Build history of the part. All positions in model axes, mm. A direction names the side the tool comes from. Give positions to 0.01 mm unless a question says otherwise; leave off trailing zeros. Write each loop counter-clockwise with the first axis right and the second up, starting at its lowest first coordinate (ties: lowest second). Pieces come first, ordered by that corner, then holes. Notation, with made-up numbers: (59.25, 23.5) -> (106.25, 23.5) arc R23 cw to (106.25, 43.5) -> close; hole circle Ø7 at (4.25, 34). An arc over 180 degrees is marked (long way). Write item = value, one per line. Start each with the question number.
Q1. Saw through at B-B, the plane z = 0. Give the number of separate pieces and of enclosed holes in the cut face, then the cut area to 3 significant figures.
Q2. Mould opens along Z. For faces 1 (the face through (49, 5, -11.8)), 2 (the face through (45, 9, 6)), 3 (the face through (-29, 10, -7)) say: pulls with the +Z half, pulls with the -Z half, needs draft (parallel to the pull), parting line crosses it, or undercut.
Q3. Wall check: line 1 (Z direction, x = 19, y = 6); line 2 (Z direction, x = -8, y = 9.75); line 3 (X direction, y = 7.75, z = -10.5). Give the ranges that are in metal, low to high.
Q4. Drop flat-ended pins along their axis: P1, Ø2, axis at x = 33.5, z = -6, coming from the -Y side; P2, Ø1.8, axis at x = 59, z = -9, coming from the +Y side; P3, Ø3, axis at x = 19.5, y = 8, coming from the -Z side. Give the stop position or say it passes through.
Q5. Saw through at A-A, the plane x = -19.6. List the corners of the cut face in (y, z), then the cut area to 3 significant figures.
Q6. Tool access for faces 4 (the face through (-49, 5, 7.9)), 5 (the face through (49, 9, 0)), 6 (the face through (10, 10, 7)), 7 (the face through (53, 9, -6)), 8 (the face through (-0.3, 0, -9.8)): list every direction of +Z, -Z, +X, -X, +Y, -Y with a clear straight run to the whole face (end or side of a thin tool).
Q7. Saw through at D-D, the plane x = 61. List the corners of the cut face in (y, z).
from build123d import *

# Parameters (mm, degrees)
SKETCH3_R              = 9.4
BOSS_EXTRUDE1_DEPTH    = 10
BOSS_EXTRUDE2_START    = -1
BOSS_EXTRUDE2_DEPTH    = 1
FILLET2_R              = 2
LPATTERN1_COUNT        = 7
LPATTERN1_PITCH        = 19.6
FILLET2_OF_LPATTERN1_R = 2
FILLET3_R              = 2
SKETCH4_5_W            = 138
SKETCH4_5_H            = 8.5
CUT_EXTRUDE2_DEPTH     = 1
SKETCH4_6_W            = 8.5
SKETCH4_6_H            = 20
CUT_EXTRUDE3_DEPTH     = 1
LPATTERN2_COUNT        = 7
LPATTERN2_PITCH        = 19.6


with BuildPart() as part:
    # Sketch3 → Boss-Extrude1 (new body)
    # profile 1 of 5: a face of its own
    with BuildSketch(Plane(origin=(0, 0, 0), x_dir=(1, 0, 0), z_dir=(0, 1, 0))):
        Polygon((-69, 10), (-69, -10), (-50.537564435, -10), (-51.75, -7.9), (-46.25, -7.9), (-47.462435565, -10), (-12.537564435, -10), (-13.75, -7.9), (-8.25, -7.9), (-9.462435565, -10), (9.462435565, -10), (8.25, -7.9), (13.75, -7.9), (12.537564435, -10), (47.462435565, -10), (46.25, -7.9), (51.75, -7.9), (50.537564435, -10), (69, -10), (69, 10), (50.460769515, 10), (47.539230485, 10), (12.460769515, 10), (9.539230485, 10), (-9.539230485, 10), (-12.460769515, 10), (-47.539230485, 10), (-50.460769515, 10), align=None)
        with Locations(Location((-58.8, 0, 0), (0, 0, 270))):
            Circle(SKETCH3_R, mode=Mode.SUBTRACT)
        with Locations(Location((-39.2, 0, 0), (0, 0, 270))):
            Circle(SKETCH3_R, mode=Mode.SUBTRACT)
        with Locations(Location((-19.6, 0, 0), (0, 0, 270))):
            Circle(SKETCH3_R, mode=Mode.SUBTRACT)
        with Locations(Location((0, 0, 0), (0, 0, 270))):
            Circle(SKETCH3_R, mode=Mode.SUBTRACT)
        with Locations(Location((19.6, 0, 0), (0, 0, 270))):
            Circle(SKETCH3_R, mode=Mode.SUBTRACT)
        with Locations(Location((39.2, 0, 0), (0, 0, 270))):
            Circle(SKETCH3_R, mode=Mode.SUBTRACT)
        with Locations(Location((58.8, 0, 0), (0, 0, 270))):
            Circle(SKETCH3_R, mode=Mode.SUBTRACT)
    # profile 2 of 5: a face of its own
    with BuildSketch(Plane(origin=(0, 0, 0), x_dir=(1, 0, 0), z_dir=(0, 1, 0))):
        Polygon((-51.5, 11.8), (-50.460769515, 10), (-47.539230485, 10), (-46.5, 11.8), align=None)
    # profile 3 of 5: a face of its own
    with BuildSketch(Plane(origin=(0, 0, 0), x_dir=(1, 0, 0), z_dir=(0, 1, 0))):
        Polygon((-13.5, 11.8), (-12.460769515, 10), (-9.539230485, 10), (-8.5, 11.8), align=None)
    # profile 4 of 5: a face of its own
    with BuildSketch(Plane(origin=(0, 0, 0), x_dir=(1, 0, 0), z_dir=(0, 1, 0))):
        Polygon((8.5, 11.8), (9.539230485, 10), (12.460769515, 10), (13.5, 11.8), align=None)
    # profile 5 of 5: a face of its own
    with BuildSketch(Plane(origin=(0, 0, 0), x_dir=(1, 0, 0), z_dir=(0, 1, 0))):
        Polygon((46.5, 11.8), (47.539230485, 10), (50.460769515, 10), (51.5, 11.8), align=None)
    extrude(amount=BOSS_EXTRUDE1_DEPTH)

    # Sketch4 → Boss-Extrude2 (add)
    with BuildSketch(Plane(origin=(0, 10, 0), x_dir=(1, 0, 0), z_dir=(0, 1, 0)).offset(BOSS_EXTRUDE2_START)):
        with BuildLine():
            Line((54.55, 4.25), (54.55, 8.384360441))
            ThreePointArc((54.55, 8.384360441), (52.153196257, 6.646803743), (50.415639559, 4.25))
            Line((50.415639559, 4.25), (54.55, 4.25))
        make_face()
        with BuildLine():
            Line((54.55, -4.25), (50.415639559, -4.25))
            ThreePointArc((50.415639559, -4.25), (52.153196257, -6.646803743), (54.55, -8.384360441))
            Line((54.55, -8.384360441), (54.55, -4.25))
        make_face()
        with BuildLine():
            Line((67.184360441, -4.25), (63.05, -4.25))
            Line((63.05, -4.25), (63.05, -8.384360441))
            ThreePointArc((63.05, -8.384360441), (65.446803743, -6.646803743), (67.184360441, -4.25))
        make_face()
        with BuildLine():
            ThreePointArc((67.184360441, 4.25), (65.446803743, 6.646803743), (63.05, 8.384360441))
            Line((63.05, 8.384360441), (63.05, 4.25))
            Line((63.05, 4.25), (67.184360441, 4.25))
        make_face()
    boss_extrude2 = extrude(amount=BOSS_EXTRUDE2_DEPTH)

    # Fillet2
    fillet2_edges = [part.edges().sort_by_distance(p)[0] for p in [
        (54.55, 9.5, -4.25),
        (54.55, 9.5, 4.25),
        (63.05, 9.5, 4.25),
        (63.05, 9.5, -4.25),
    ]]
    fillet(fillet2_edges, radius=FILLET2_R)

    # LPattern1: Boss-Extrude2 ×7
    with Locations(*[(-i * LPATTERN1_PITCH, 0, 0) for i in range(1, LPATTERN1_COUNT)]):
        add(boss_extrude2)

    # Fillet2 of LPattern1
    fillet2_of_lpattern1_edges = [part.edges().sort_by_distance(p)[0] for p in [
        (34.95, 9.5, -4.25),
        (34.95, 9.5, 4.25),
        (43.45, 9.5, 4.25),
        (43.45, 9.5, -4.25),
        (15.35, 9.5, -4.25),
        (15.35, 9.5, 4.25),
        (23.85, 9.5, 4.25),
        (23.85, 9.5, -4.25),
        (-4.25, 9.5, -4.25),
        (-4.25, 9.5, 4.25),
        (4.25, 9.5, 4.25),
        (4.25, 9.5, -4.25),
        (-23.85, 9.5, -4.25),
        (-23.85, 9.5, 4.25),
        (-15.35, 9.5, 4.25),
        (-15.35, 9.5, -4.25),
        (-43.45, 9.5, -4.25),
        (-43.45, 9.5, 4.25),
        (-34.95, 9.5, 4.25),
        (-34.95, 9.5, -4.25),
        (-63.05, 9.5, -4.25),
        (-63.05, 9.5, 4.25),
        (-54.55, 9.5, 4.25),
        (-54.55, 9.5, -4.25),
    ]]
    fillet(fillet2_of_lpattern1_edges, radius=FILLET2_OF_LPATTERN1_R)

    # Fillet3
    fillet3_edges = [part.edges().sort_by_distance(p)[0] for p in [
        (-69, 5, 10),
        (-69, 5, -10),
        (69, 5, -10),
        (69, 5, 10),
    ]]
    fillet(fillet3_edges, radius=FILLET3_R)

    # Sketch4_5 → Cut-Extrude2 (cut)
    with BuildSketch(Plane(origin=(0, 10, 0), x_dir=(1, 0, 0), z_dir=(0, 1, 0))):
        Rectangle(SKETCH4_5_W, SKETCH4_5_H)
    extrude(amount=-CUT_EXTRUDE2_DEPTH, mode=Mode.SUBTRACT)

    # Sketch4_6 → Cut-Extrude3 (cut)
    with BuildSketch(Plane(origin=(0, 10, 0), x_dir=(1, 0, 0), z_dir=(0, 1, 0))):
        with Locations((58.8, 0)):
            Rectangle(SKETCH4_6_W, SKETCH4_6_H)
    cut_extrude3 = extrude(amount=-CUT_EXTRUDE3_DEPTH, mode=Mode.SUBTRACT)

    # LPattern2: Cut-Extrude3 ×7
    with Locations(*[(-i * LPATTERN2_PITCH, 0, 0) for i in range(1, LPATTERN2_COUNT)]):
        add(cut_extrude3, mode=Mode.SUBTRACT)


solid = part.part
Report:
q1.separate_pieces = 8
q1.enclosed_holes = 0
q1.area = 57.6 mm2
q2.face_1 = pulls with the -Z half
q2.face_2 = undercut
q2.face_3 = needs draft
q3.line_1 = -10 to -9.38, 9.38 to 10
q3.line_2 = -10 to -4.25, 4.25 to 10
q3.line_3 = -50.75 to -47.25, -12.75 to -9.25, 9.25 to 12.75, 47.25 to 50.75
q4.P1 = 9
q4.P2 = 9
q4.P3 = -10
q5.outline = (0, -10) -> (9, -10) -> (9, -9.4) -> (0, -9.4) -> close; (0, 9.4) -> (9, 9.4) -> (9, 10) -> (0, 10) -> close
q5.area = 10.8 mm2
q6.face_4 = +Y, -Y
q6.face_5 = +X, -X, +Y
q6.face_6 = +Z, -Z, +X, -X, +Y
q6.face_7 = -Y
q6.face_8 = +Z, -Z, +X, -X, -Y
q7.outline = (0, -10) -> (9, -10) -> (9, -9.14) -> (0, -9.14) -> close; (0, 9.14) -> (9, 9.14) -> (9, 10) -> (0, 10) -> close
